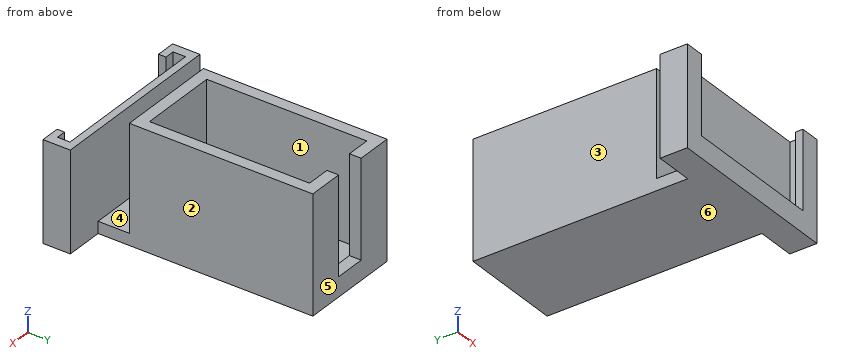
from build123d import *

# Parameters (mm, degrees)
SKETCH1_W           = 20.31
SKETCH1_H           = 41
BOSS_EXTRUDE1_DEPTH = 3
SKETCH2_W           = 26.31
SKETCH2_H           = 47
SKETCH2_W_2         = 20.31
SKETCH2_H_2         = 41
BOSS_EXTRUDE2_DEPTH = 5
SKETCH3_W           = 26.31
SKETCH3_H           = 8
BOSS_EXTRUDE3_DEPTH = 3
SKETCH4_W           = 46
SKETCH4_H           = 1.9
BOSS_EXTRUDE4_DEPTH = 5.5
SKETCH5_W           = 46
SKETCH5_H           = 3.2
BOSS_EXTRUDE5_DEPTH = 3
BOSS_EXTRUDE6_DEPTH = 5
SKETCH8_W           = 2.5
SKETCH8_H           = 3.2
BOSS_EXTRUDE7_DEPTH = 2.5
BOSS_EXTRUDE8_DEPTH = 20
BOSS_EXTRUDE9_DEPTH = 20


with BuildPart() as part:
    # Sketch1 → Boss-Extrude1 (new body)
    with BuildSketch(Plane.XY):
        Rectangle(SKETCH1_W, SKETCH1_H)
    extrude(amount=BOSS_EXTRUDE1_DEPTH)

    # Sketch2 → Boss-Extrude2 (add)
    with BuildSketch(Plane(origin=(0, 0, 0), x_dir=(-1, 0, 0), z_dir=(0, 0, -1))):
        Rectangle(SKETCH2_W, SKETCH2_H)
        Rectangle(SKETCH2_W_2, SKETCH2_H_2, mode=Mode.SUBTRACT)
    extrude(amount=-BOSS_EXTRUDE2_DEPTH)

    # Sketch3 → Boss-Extrude3 (add)
    with BuildSketch(Plane(origin=(0, 0, 0), x_dir=(-1, 0, 0), z_dir=(0, 0, -1))):
        with Locations((0, -27.5)):
            Rectangle(SKETCH3_W, SKETCH3_H)
    extrude(amount=-BOSS_EXTRUDE3_DEPTH)

    # Sketch4 → Boss-Extrude4 (add)
    with BuildSketch(Plane(origin=(0, 0, 0), x_dir=(-1, 0, 0), z_dir=(0, 0, -1))):
        with Locations((0, -37.55)):
            Rectangle(SKETCH4_W, SKETCH4_H)
        Polygon((13.155, -31.5), (0, -31.5), (-13.155, -31.5), (-23, -31.5), (-23, -33.4), (23, -33.4), (23, -31.5), align=None)
    extrude(amount=-BOSS_EXTRUDE4_DEPTH)


with BuildPart() as boss_extrude4_piece_1:
    # of the separate pieces the step leaves, piece 1, a body of its own (boss_extrude4_pieces)
    add(part.part.solids().sort_by_distance((-13.155, -31.5, 0))[0])



with BuildPart() as boss_extrude4_piece_2:
    # of the separate pieces the step leaves, piece 2, a body of its own (boss_extrude4_pieces)
    add(part.part.solids().sort_by_distance((-23, -38.5, 0))[0])


with BuildPart() as boss_extrude4_piece_1_1:
    add(boss_extrude4_piece_1.part)

    add(boss_extrude4_piece_2.part)  # Boss-Extrude5 merges Boss-Extrude4 piece 2
    # Sketch5 → Boss-Extrude5 (add)
    with BuildSketch(Plane(origin=(0, 0, 0), x_dir=(-1, 0, 0), z_dir=(0, 0, -1))):
        with Locations((0, -35)):
            Rectangle(SKETCH5_W, SKETCH5_H)
    extrude(amount=-BOSS_EXTRUDE5_DEPTH)

    # Sketch6 → Boss-Extrude6 (add)
    with BuildSketch(Plane.XY.offset(5)):
        Polygon((4.010497469, 23.5), (4.010497469, 20.5), (10.155, 20.5), (10.155, -20.5), (-10.155, -20.5), (-10.155, 20.5), (-3.989502531, 20.5), (-3.989502531, 23.5), (-13.155, 23.5), (-13.155, -23.5), (13.155, -23.5), (13.155, 23.5), align=None)
    extrude(amount=BOSS_EXTRUDE6_DEPTH)

    # Sketch8 → Boss-Extrude7 (add)
    with BuildSketch(Plane.XY.offset(3)):
        with Locations((-21.75, -35)):
            Rectangle(SKETCH8_W, SKETCH8_H)
        with Locations((21.75, -35)):
            Rectangle(SKETCH8_W, SKETCH8_H)
    extrude(amount=BOSS_EXTRUDE7_DEPTH)

    # Sketch9 → Boss-Extrude8 (add)
    with BuildSketch(Plane.XY.offset(5.5)):
        Polygon((-23, -31.5), (-23, -38.5), (-18, -38.5), (-18, -36.6), (-20.5, -36.6), (-20.5, -33.4), (20.5, -33.4), (20.5, -36.6), (18, -36.6), (18, -38.5), (23, -38.5), (23, -31.5), align=None)
    extrude(amount=BOSS_EXTRUDE8_DEPTH)

    # Sketch12 → Boss-Extrude9 (add)
    with BuildSketch(Plane.XY.offset(10)):
        Polygon((13.155, -23.5), (13.155, 23.5), (4.010497469, 23.5), (4.010497469, 20.5), (10.155, 20.5), (10.155, -20.5), (-10.155, -20.5), (-10.155, 20.5), (-3.989502531, 20.5), (-3.989502531, 23.5), (-13.155, 23.5), (-13.155, -23.5), align=None)
    extrude(amount=BOSS_EXTRUDE9_DEPTH)


solid = boss_extrude4_piece_1_1.part
Work out the finished part from the listing and answer in its coordinate system (mm). Face numbers are marked on the shaded views. A direction names the side the tool comes from. Give positions to 0.01 mm unless a question says otherwise; leave off trailing zeros. Order: outer loops, then holes, each group sorted by start corner. A loop starts at its lowest first (then second) coordinate and runs counter-clockwise, first axis right, second up. Notation, with made-up numbers: (70, -16.75) -> (84, -16.75) arc R17 ccw to (84, -12.75) -> close; hole circle Ø9 at (38.25, 40). An arc over 180 degrees is marked (long way). Answer as a JSON object with one key per item and string values. Group by question number.
1. A tool of negligible diameter and unlimited length cuts with its end or side. For the marked faces 1, 2 and 3, from which of +Z, -Z, +X, -X, +Y, -Y can it reach the whole face along a straight path? Write none if from no direction.
2. Section D-D on z = 26.75 is taken. Determine the outline of the cut face in (x, y) (1 decimal), plus the area to 3 significant figures.
3. The mould has two halves that part along Y. Classify the marked faces 4, 5 and 6: released by +Y, released by -Y, zero draft, split by the parting line, or undercut.
4. Consider line 1 along Y through (x, z) = (-10, 6.5); line 2 along X through (y, z) = (3.5, 7.25) (3 decimals); line 3 along Y through (x, z) = (-9, 25.75). Determine where each line is inside the solid, lowest interval first. Write a range as [from, to].
5. Section B-B on x = -2 is taken. Determine the outline of the cut face in (y, z), plus the area to 4 significant figures.
6. Section A-A on z = 22.5 is taken. Determine the outline of the cut face in (x, y) (1 decimal).
7. Section C-C on y = -19 is taken. Determine the outline of the cut face in (x, z) (3 decimals).
8. Flat-ended cylindrical pins translate along their axes: pin 1 Ø2.5 at (x, y) = (6.5, -35.5) entering from +Z; pin 2 Ø12 at (y, z) = (14, 7) entering from +X (3 decimals); pin 3 Ø1 at (x, z) = (-16, 5.5) entering from +Y. Find the tip coordinate at first contact, or state that the pin passes through.
Result sheet:
{
 "1": {"face 1": "+Z", "face 2": "+Z, -Z, +X, +Y", "face 3": "+Z, -Z, -X, +Y"},
 "2": {"outline": "(-13.2, -23.5) -> (13.2, -23.5) -> (13.2, 23.5) -> (4, 23.5) -> (4, 20.5) -> (10.2, 20.5) -> (10.2, -20.5) -> (-10.2, -20.5) -> (-10.2, 20.5) -> (-4, 20.5) -> (-4, 23.5) -> (-13.2, 23.5) -> close", "area": "380 mm^2"},
 "3": {"face 4": "undercut", "face 5": "released by +Y", "face 6": "zero draft"},
 "4": {"line 1": "y = [-33.4, -31.5], [-23.5, -20.5], [20.5, 23.5]", "line 2": "x = [-13.155, -10.155], [10.155, 13.155]", "line 3": "y = [-23.5, -20.5], [20.5, 23.5]"},
 "5": {"outline": "(-38.5, 0) -> (23.5, 0) -> (23.5, 5) -> (20.5, 5) -> (20.5, 3) -> (-20.5, 3) -> (-20.5, 30) -> (-23.5, 30) -> (-23.5, 3) -> (-31.5, 3) -> (-31.5, 25.5) -> (-33.4, 25.5) -> (-33.4, 3) -> (-36.6, 3) -> (-36.6, 5.5) -> (-38.5, 5.5) -> close", "area": "320.5 mm^2"},
 "6": {"outline": "(-23, -38.5) -> (-18, -38.5) -> (-18, -36.6) -> (-20.5, -36.6) -> (-20.5, -33.4) -> (20.5, -33.4) -> (20.5, -36.6) -> (18, -36.6) -> (18, -38.5) -> (23, -38.5) -> (23, -31.5) -> (-23, -31.5) -> close; (-13.2, -23.5) -> (13.2, -23.5) -> (13.2, 23.5) -> (4, 23.5) -> (4, 20.5) -> (10.2, 20.5) -> (10.2, -20.5) -> (-10.2, -20.5) -> (-10.2, 20.5) -> (-4, 20.5) -> (-4, 23.5) -> (-13.2, 23.5) -> close"},
 "7": {"outline": "(-13.155, 0) -> (13.155, 0) -> (13.155, 30) -> (10.155, 30) -> (10.155, 3) -> (-10.155, 3) -> (-10.155, 30) -> (-13.155, 30) -> close"},
 "8": {"pin 1": "stops at z = 5.5", "pin 2": "stops at x = 13.155", "pin 3": "stops at y = -31.5"}
}
